Here's how the part is built. I have some questions about the finished solid (model axes, mm). Face numbers are marked on the shaded views. Round coordinates to 2 decimals unless told otherwise and drop trailing zeros. Write each loop counter-clockwise with the first axis right and the second up, starting at its lowest first coordinate (ties: lowest second). Pieces come first, ordered by that corner, then holes. Notation, with made-up numbers: (79.25, 28) -> (138.25, 28) arc R30 cw to (138.25, 59) -> close; hole circle Ø8 at (30.25, -27.5). An arc over 180 degrees is marked (long way). Put each result on its own line as item: value. Start each with the question number.
1) We'd pull the mould along Y, two halves only. Please class the marked faces 1, 2, 3 and 4: released by +Y, released by -Y, zero draft, split by the parting line, or undercut.
2) If I drill on line 1 along Y through (x, z) = (0, 3.65); line 2 along X through (y, z) = (8, 3); line 3 along Z through (x, y) = (2.35, 7.5), over which ranges is the centre line in solid material (lowest first)? Write a range as [from, to].
3) I want a section at B-B, the plane y = 7.5. List the corners of the cut face in (x, z) for me.
4) I want a section at A-A, the plane x = 0. List the corners of the cut face in (y, z) for me.
5) Will these pins go through, and if not, where does the flat tip stop? P1, Ø2, axis at x = -4, z = 2.5, coming from the +Y side; P2, Ø4.5, axis at x = -3, y = 18.5, coming from the +Z side; P3, Ø3, axis at x = -1.5, y = 42, coming from the -Z side.
6) I want a section at D-D, the plane y = 35.5. List the corners of the cut face in (x, z) for me, then the cut area to 3 significant figures.
7) I want a section at C-C, the plane z = 1.5. List the corners of the cut face in (x, y) for me, then the cut area to 3 significant figures.
from build123d import *

# Parameters (mm, degrees)
EXTRUDE_1_DEPTH     = 4
CUT_EXTRUDE_1_DEPTH = 3
SKETCH_5_R          = 1.25
CUT_EXTRUDE_2_DEPTH = 12.4
SKETCH_6_W          = 1
SKETCH_6_H          = 10
CUT_EXTRUDE_3_DEPTH = 16.3
SKETCH_9_W          = 5
SKETCH_9_H          = 10
EXTRUDE_4_DEPTH     = 3
SKETCH_10_R         = 1.1
CUT_EXTRUDE_4_DEPTH = 5.1


with BuildPart() as part:
    # 草圖1 → 填料-伸長1 (new body)
    with BuildSketch(Plane.XY):
        with BuildLine():
            Line((7.5, 0), (7.5, 52))
            ThreePointArc((7.5, 52), (0, 59.5), (-7.5, 52))
            Line((-7.5, 52), (-7.5, 0))
            Line((-7.5, 0), (7.5, 0))
        make_face()
    extrude(amount=EXTRUDE_1_DEPTH)

    # 草圖3 → 除料-伸長1 (cut)
    with BuildSketch(Plane.XY):
        with BuildLine():
            ThreePointArc((-2.296635758, 50), (0, 52.296635758), (2.296635758, 50))
            Line((2.296635758, 50), (5, 33.5))
            Line((5, 33.5), (2.272331993, 16.632537074))
            ThreePointArc((2.272331993, 16.632537074), (-0.184323371, 14.705540024), (-2.301851795, 17))
            Line((-2.301851795, 17), (-5, 33.5))
            Line((-5, 33.5), (-2.296635758, 50))
        make_face()
    extrude(amount=CUT_EXTRUDE_1_DEPTH, mode=Mode.SUBTRACT)

    # 草圖5 → 除料-伸長2 (cut)
    with BuildSketch(Plane.XY):
        with Locations((0, 33.5)):
            Circle(SKETCH_5_R)
    extrude(amount=CUT_EXTRUDE_2_DEPTH, mode=Mode.SUBTRACT)

    # 草圖6 → 除料-伸長3 (cut)
    with BuildSketch(Plane.XY):
        with Locations((0, 5)):
            Rectangle(SKETCH_6_W, SKETCH_6_H)
    extrude(amount=CUT_EXTRUDE_3_DEPTH, mode=Mode.SUBTRACT)

    # 草圖9 → 填料-伸長4 (add)
    with BuildSketch(Plane(origin=(0.5, 0, 0), x_dir=(0, 0, -1), z_dir=(1, 0, 0))):
        with Locations((-6.46178466, 5)):
            Rectangle(SKETCH_9_W, SKETCH_9_H)
    extrude(amount=EXTRUDE_4_DEPTH)

    # 草圖10 → 除料-伸長4 (cut)
    with BuildSketch(Plane(origin=(0.5, 0, 0), x_dir=(0, 0, -1), z_dir=(1, 0, 0))):
        with Locations((-6.48089233, 7.5)):
            Circle(SKETCH_10_R)
        with Locations((-6.48089233, 2.5)):
            Circle(SKETCH_10_R)
    extrude(amount=CUT_EXTRUDE_4_DEPTH, mode=Mode.SUBTRACT)


solid = part.part
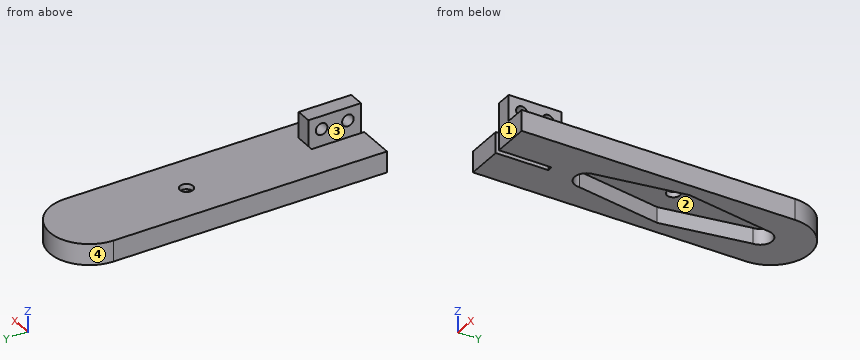
Findings:
1. face 1: released by -Y
1. face 2: undercut
1. face 3: zero draft
1. face 4: released by +Y
2. line 1: y = [10, 32.25], [34.75, 59.5]
2. line 2: x = [-7.5, -0.5], [0.5, 7.5]
2. line 3: z = [0, 5.38], [7.58, 8.96]
3. outline: (-7.5, 0) -> (-0.5, 0) -> (-0.5, 4) -> (-7.5, 4) -> close; (0.5, 0) -> (7.5, 0) -> (7.5, 4) -> (3.5, 4) -> (3.5, 5.38) -> (0.5, 5.38) -> close; (0.5, 7.58) -> (3.5, 7.58) -> (3.5, 8.96) -> (0.5, 8.96) -> close
4. outline: (10, 0) -> (14.7, 0) -> (14.7, 3) -> (32.25, 3) -> (32.25, 4) -> (10, 4) -> close; (34.75, 3) -> (52.3, 3) -> (52.3, 0) -> (59.5, 0) -> (59.5, 4) -> (34.75, 4) -> close
5. P1: stops at y = 58.87
5. P2: stops at z = 4
5. P3: stops at z = 3
6. outline: (-7.5, 0) -> (-4.67, 0) -> (-4.67, 3) -> (4.67, 3) -> (4.67, 0) -> (7.5, 0) -> (7.5, 4) -> (-7.5, 4) -> close
6. area: 32.0 mm2
7. outline: (-7.5, 0) -> (-0.5, 0) -> (-0.5, 10) -> (0.5, 10) -> (0.5, 0) -> (7.5, 0) -> (7.5, 52) arc R7.5 ccw to (-7.5, 52) -> close; hole (-5, 33.5) -> (-2.3, 17) arc R2.3 ccw to (2.27, 16.63) -> (5, 33.5) -> (2.3, 50) arc R2.3 ccw to (-2.3, 50) -> close
7. area: 601 mm2
